Verification items for the finished model (mm, model axes). A direction names the side the tool comes from. Coordinates: 2 decimals unless noted, no trailing zeros. Order: outer loops, then holes, each group sorted by start corner. A loop starts at its lowest first (then second) coordinate and runs counter-clockwise, first axis right, second up. Notation, with made-up numbers: M 88.5,9.5 L 93.5,9.5 A22 cw 93.5,15.5 Z; hole C 48.25,-29.75 d4. An arc over 180 degrees is marked long. Answer as a JSON object with one key per item and string values. Group by question number.
(1) Gauge pin test, flat ends, axial feed: pin 1 Ø4 at (x, z) = (42.5, 70) entering from +Y; pin 2 Ø1.7 at (x, y) = (-7, 1) entering from +Z. Record the tip position at first contact, or that the pin passes through.
(2) Material ranges on line 1 (X direction, y = 0.9, z = 70); line 2 (X direction, y = 0.9, z = 80); line 3 (Z direction, x = -42.5, y = 0.8), recorded low to high.
(3) Mould release check, pull along Z, two halves, no side actions. Record for faces 4 (the face through (17.5, 2, -87)), 5 (the face through (-34, 2, 100)), 6 (the face through (-34, 2, -100)), 7 (the face through (41.15, 1.72, -68.97)): released by +Z, released by -Z, zero draft, split by the parting line, or undercut.
(4) Access from +Z, -Z, +X, -X, +Y, -Y to the whole of each face (thin tool, end or side, straight path). Record for faces 1 (the face through (0, 2, 75)), 2 (the face through (-17.5, 2, 0)), 3 (the face through (-17.5, 2, -87)).
(5) Cross-section at B-B (x = -11). Enter the section's corners in (y, z).
(6) Cross-section at A-A (y = 1.35). Count the separate pieces of the cut face and the enclosed holes in it, plus the area to 3 significant figures.
from build123d import *

# Parameters (mm, degrees)
CROQUIS1_W              = 100
CROQUIS1_H              = 200
SALIENTE_EXTRUIR1_DEPTH = 3.4
CROQUIS2_R              = 1.7
CROQUIS2_W              = 35
CROQUIS2_H              = 25
CROQUIS2_H_2            = 50
CORTAR_EXTRUIR1_DEPTH   = 3.4


with BuildPart() as part:
    # Croquis1 → Saliente-Extruir1 (new body)
    with BuildSketch(Plane(origin=(0, 0, 0), x_dir=(1, 0, 0), z_dir=(0, 1, 0))):
        Rectangle(CROQUIS1_W, CROQUIS1_H)
    extrude(amount=SALIENTE_EXTRUIR1_DEPTH)

    # Croquis2 → Cortar-Extruir1 (cut)
    with BuildSketch(Plane(origin=(0, 3.4, 0), x_dir=(1, 0, 0), z_dir=(0, 1, 0))):
        with Locations((42.5, -80)):
            Circle(CROQUIS2_R)
        with Locations((42.5, -70)):
            Circle(CROQUIS2_R)
        with Locations((-42.5, -80)):
            Circle(CROQUIS2_R)
        with Locations((-42.5, -70)):
            Circle(CROQUIS2_R)
        with Locations((42.5, 70)):
            Circle(CROQUIS2_R)
        with Locations((42.5, 80)):
            Circle(CROQUIS2_R)
        with Locations((-42.5, 70)):
            Circle(CROQUIS2_R)
        with Locations((-42.5, 80)):
            Circle(CROQUIS2_R)
        with Locations((0, 87.5)):
            Rectangle(CROQUIS2_W, CROQUIS2_H)
        Rectangle(CROQUIS2_W, CROQUIS2_H_2)
        with Locations((0, -87.5)):
            Rectangle(CROQUIS2_W, CROQUIS2_H)
    extrude(amount=-CORTAR_EXTRUIR1_DEPTH, mode=Mode.SUBTRACT)


solid = part.part
Taken from the geometry:
{
 "1": {"pin 1": "stops at y = 3.4", "pin 2": "stops at z = 75"},
 "2": {"line 1": "x = -50 to -44.2, -40.8 to 40.8, 44.2 to 50", "line 2": "x = -50 to -44.2, -40.8 to -17.5, 17.5 to 40.8, 44.2 to 50", "line 3": "z = -100 to -81.7, -78.3 to -71.7, -68.3 to 68.3, 71.7 to 78.3, 81.7 to 100"},
 "3": {"face 4": "zero draft", "face 5": "released by +Z", "face 6": "released by -Z", "face 7": "undercut"},
 "4": {"face 1": "+Z, +Y, -Y", "face 2": "+Y, -Y", "face 3": "-Z, +Y, -Y"},
 "5": {"outline": "M 0,-75 L 3.4,-75 L 3.4,-25 L 0,-25 Z; M 0,25 L 3.4,25 L 3.4,75 L 0,75 Z"},
 "6": {"separate pieces": "1", "enclosed holes": "9", "area": "16,400 mm²"}
}
